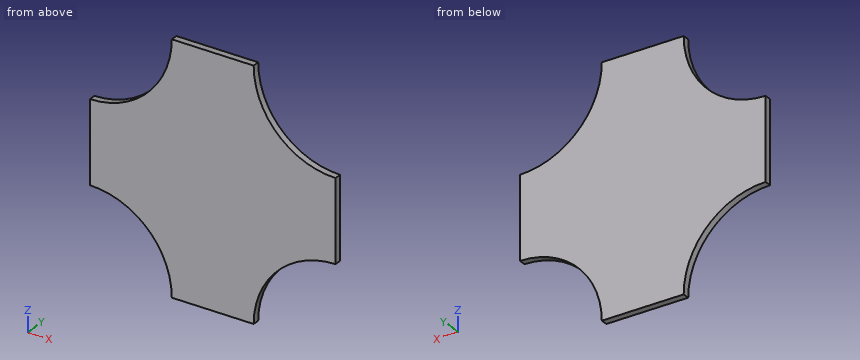
```python
from build123d import *

# Parameters (mm, degrees)
BOSS_EXTRUDE1_DEPTH = 10


with BuildPart() as part:
    # Sketch1 → Boss-Extrude1 (new body)
    with BuildSketch(Plane(origin=(0, 0, 0), x_dir=(1, 0, 0), z_dir=(0, 1, 0))):
        Polygon((60, -60), (60, -180), (-60, -180), (-60, -60), (-180, -60), (-180, 60), (-60, 60), (-60, 180), (60, 180), (60, 60), (180, 60), (180, -60), align=None)
        with BuildLine():
            Line((-60, 180), (-60, 60))
            Line((-60, 60), (-180, 60))
            ThreePointArc((-180, 60), (-95.147186258, 95.147186258), (-60, 180))
        make_face()
        with BuildLine():
            ThreePointArc((60, 180), (95.147186258, 95.147186258), (180, 60))
            Line((180, 60), (60, 60))
            Line((60, 60), (60, 180))
        make_face()
        with BuildLine():
            ThreePointArc((180, -60), (95.147186258, -95.147186258), (60, -180))
            Line((60, -180), (60, -60))
            Line((60, -60), (180, -60))
        make_face()
        with BuildLine():
            Line((-180, -60), (-60, -60))
            Line((-60, -60), (-60, -180))
            ThreePointArc((-60, -180), (-95.147186258, -95.147186258), (-180, -60))
        make_face()
    extrude(amount=BOSS_EXTRUDE1_DEPTH)


solid = part.part
```
Geometry check sheet. Reference: the model listing, model coordinates, mm. Give positions to 0.01 mm unless a question says otherwise; leave off trailing zeros. Order: outer loops, then holes, each group sorted by start corner. A loop starts at its lowest first (then second) coordinate and runs counter-clockwise, first axis right, second up. Notation, with made-up numbers: (-6, 56) - (47, 56) arc R14 ccw to (47, 61) - close; hole circle Ø3 at (9.5, 76.5). An arc over 180 degrees is marked (long way). Write item = value, one per line. Start each with the question number.
1) Scan lines: L1, parallel to X at y = 2, z = -106; L2, parallel to Z at x = 149, y = 6.75; L3, parallel to X at y = 3, z = 134.5. Record each from-to range of solid material in increasing order.
2) Gauge pin test, flat end, axial feed: pin 1 Ø4 at (x, y) = (83, 8) entering from -Z. Record the tip position at first contact, or that the pin passes through.
3) Section check A-A (y = 3.5). Enter the section's corners in (x, z), then the cut area to 3 significant figures.
4) Section check C-C (x = -107). Enter the section's corners in (y, z).
5) Section check B-B (z = -144.5). Enter the section's corners in (x, y), then the cut area to 3 significant figures.
Geometry check:
q1.L1 = -85.53 to 85.53
q1.L2 = -64.07 to 64.07
q1.L3 = -68.96 to 68.96
q2.pin_1 = -112.18
q3.outline = (-180, -60) arc R120 cw to (-60, -180) - (60, -180) arc R120 cw to (180, -60) - (180, 60) arc R120 cw to (60, 180) - (-60, 180) arc R120 cw to (-180, 60) - close
q3.area = 84,400 mm2
q4.outline = (0, -84.76) - (10, -84.76) - (10, 84.76) - (0, 84.76) - close
q5.outline = (-65.37, 0) - (65.37, 0) - (65.37, 10) - (-65.37, 10) - close
q5.area = 1,310 mm2
